Can you work these out from the drawing? Everything is in mm from the part's minimum corner. A direction names the side the tool comes from. Coordinates: 2 decimals unless noted, no trailing zeros. Order: outer loops, then holes, each group sorted by start corner. A loop starts at its lowest first (then second) coordinate and runs counter-clockwise, first axis right, second up. Notation, with made-up numbers: (-17, 14) - (-7, 14) arc R23 ccw to (-7, 36) - close; hole circle Ø5 at (8.5, 56). An arc over 180 degrees is marked (long way). Use a Markdown table: item, result. Add a question column.
(1) I want a section at A-A (x = 33.5). List the corners of the cut face in (y, z) for me.
(2) We'd pull the mould along Z, two halves only. Please class the marked faces 4, 5 and 6: pulls with the +Z half, pulls with the -Z half, needs draft (parallel to the pull), parting line crosses it, or undercut.
(3) On a 3-axis mill with a long thin cutter (end or side, diameter ignored), from which of +Z, -Z, +X, -X, +Y, -Y can I reach the whole of each face in a straight line? I mean the marked faces 1, 2 and 3. Say none if no direction works.
(4) I want a section at B-B (z = 23). List the corners of the cut face in (x, y) for me (1 decimal).
(5) If I drill on L1, parallel to X at y = 4.5, z = 20.5 (1 decimal); L2, parallel to Z at x = 21.5, y = 0.75; L3, parallel to X at y = 4, z = 14 (1 decimal), over which ranges is the centre line in solid material (lowest first)? Write a range as [from, to].
(6) I want a section at D-D (x = 6). List the corners of the cut face in (y, z) for me.
(7) I want a section at C-C (y = 4). State how many separate pieces and enclosed holes the cut face has.
(8) For pin 1 Ø2.5 at (x, z) = (35, 39.5) entering from +Y; pin 2 Ø12 at (x, z) = (29, 24.5) entering from +Y; pin 3 Ø3 at (x, y) = (28.5, 2.5) entering from -Z; pin 4 Ø2 at (y, z) = (0.5, 24) entering from -X, each with a flat end and sliding along its axis, tell me the tip position at first contact or that it passes through.
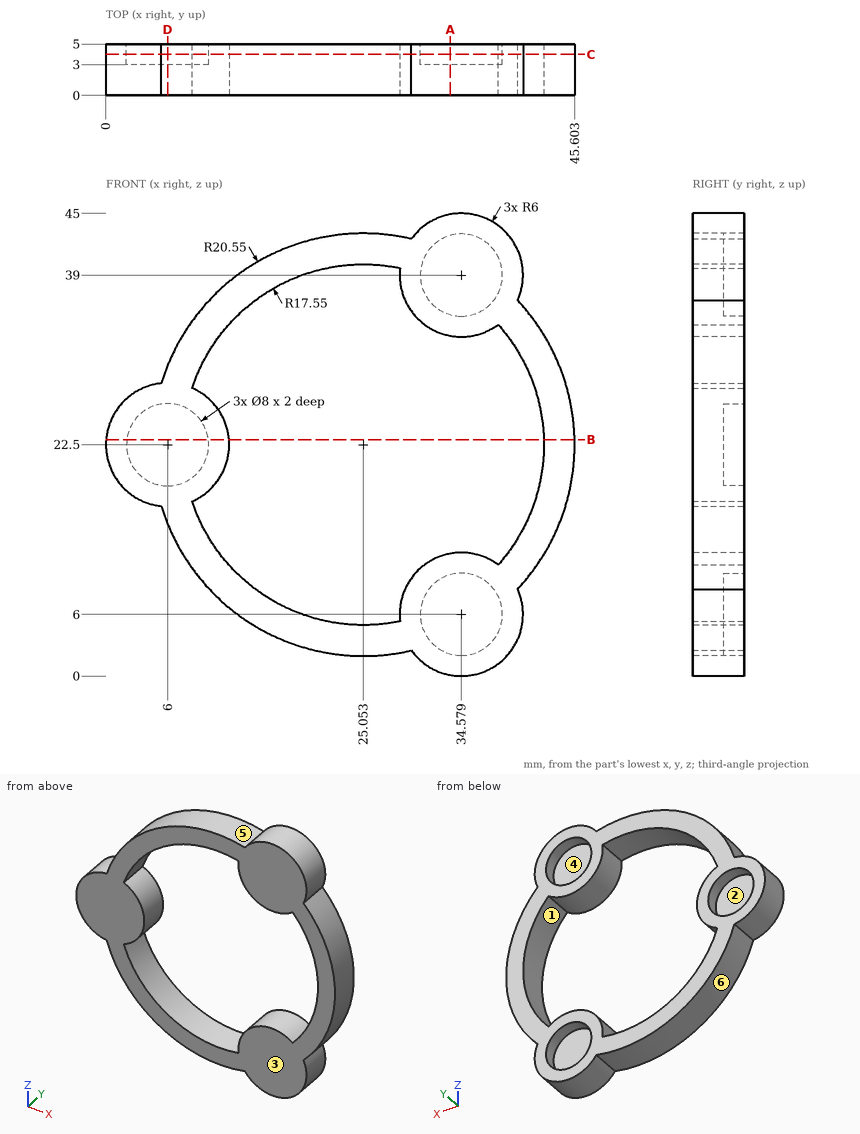
Answers follow:
| question | item | result |
|---|---|---|
| 1 | outline | (0, 0.1) - (5, 0.1) - (5, 2.15) - (3, 2.15) - (3, 9.85) - (5, 9.85) - (5, 11.9) - (0, 11.9) - close; (0, 33.1) - (5, 33.1) - (5, 35.15) - (3, 35.15) - (3, 42.85) - (5, 42.85) - (5, 44.9) - (0, 44.9) - close |
| 2 | face 4 | undercut |
| 2 | face 5 | pulls with the +Z half |
| 2 | face 6 | pulls with the -Z half |
| 3 | face 1 | +Y, -Y |
| 3 | face 2 | +Y |
| 3 | face 3 | +Z, -Z, +X, -X, -Y |
| 4 | outline | (0, 0) - (12, 0) - (12, 5) - (10, 5) - (10, 3) - (2, 3) - (2, 5) - (0, 5) - close; (42.6, 0) - (45.6, 0) - (45.6, 5) - (42.6, 5) - close |
| 5 | L1 | x = [0.3, 2.5], [9.5, 11.7], [42.5, 45.5] |
| 5 | L2 | z = [2.26, 5.31], [39.69, 42.74] |
| 5 | L3 | x = [6.3, 9.7], [40.4, 43.8] |
| 6 | outline | (0, 14.8) - (5, 14.8) - (5, 18.5) - (3, 18.5) - (3, 26.5) - (5, 26.5) - (5, 30.2) - (0, 30.2) - close |
| 7 | separate pieces | 1 |
| 7 | enclosed holes | 4 |
| 8 | pin 1 | stops at y = 3 |
| 8 | pin 2 | passes through |
| 8 | pin 3 | stops at z = 2.04 |
| 8 | pin 4 | stops at x = 0.02 |
